Design review of the part built by this model. Coordinates are the model's own, in mm. Face numbers are marked on the shaded views. A direction names the side the tool comes from. Coordinates: 2 decimals unless noted, no trailing zeros. Write each loop counter-clockwise with the first axis right and the second up, starting at its lowest first coordinate (ties: lowest second). Pieces come first, ordered by that corner, then holes. Notation, with made-up numbers: (27, -21.75) -> (75, -21.75) arc R13 cw to (75, -11.75) -> close; hole circle Ø7 at (0, -40). An arc over 180 degrees is marked (long way). Answer in a Markdown table with one row per item. Add a question column.
Item 1: Take a section at B-B, the plane y = -6. Write out the cut boundary in (x, z), and give its area (3 significant figures).
Item 2: For the marked faces 1, 2, 3 and 4, list the 3-axis set-ups (+Z, -Z, +X, -X, +Y, -Y) from which the entire face can be reached by the end or side of a thin tool; tool diameter is ignored.
Item 3: Take a section at D-D, the plane z = 2. Write out the cut boundary in (x, y), and give its area (3 significant figures).
Item 4: Clearance check with flat-ended pins moving along their axes: P1, Ø3.5, axis at y = -15, z = -3.5, coming from the +X side; P2, Ø2, axis at x = -10, z = -6.5, coming from the +Y side; P3, Ø4, axis at y = -0.5, z = 0.5, coming from the +X side. State where each tip first meets the part, or that it passes through.
Item 5: To check wall thickness, follow line 1 (Z direction, x = -5.5, y = -11); line 2 (Y direction, x = -10, z = -5.75); line 3 (Y direction, x = 2.25, z = -8). State the ranges of each line that lie inside material, in increasing order.
Item 6: Take a section at C-C, the plane y = -12.5. Write out the cut boundary in (x, z), and give its area (3 significant figures).
Item 7: Draft analysis for pull direction Y (two halves, no side actions). For the marked faces 5, 6 and 7, state which applies: released by +Y, released by -Y, zero draft, split by the parting line, or undercut.
Item 8: Take a section at A-A, the plane z = -3. Write out the cut boundary in (x, y), and give its area (3 significant figures).
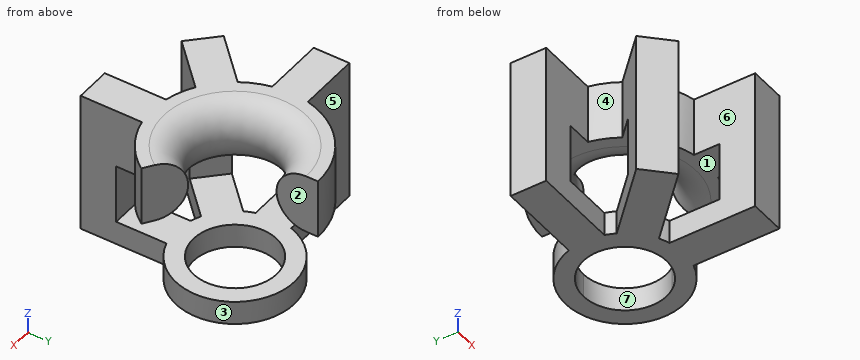
Autodesk Fusion 360 part; units mm, degrees
sketch "Sketch1" plane through (0, 0, 0) normal (1, 0, 0) x (0, 1, 0)
  line L0 (0, -2.5) -> (1, -2.5)
  line L1 (1, -2.5) -> (1, 2.5)
  line L2 (1, 2.5) -> (0, 2.5)
  arc A0 (0, 2.5) -> (0, -2.5) centre (0, 0) ccw
  line L3 (-6, 5) -> (-6, -5)
  dimension "d1" = 5
  dimension "d2" = 1
  dimension "d3" = 5
  dimension "d4" = 6
revolve "Revolve1" add sketch "Sketch1" angle 235 about axis through (0, -6, 5) along (0, 0, 1) makes body 1
sketch "Sketch2" plane through (0, 0, 2.5) normal (0, 0, 1) x (-1, 0, 0)
  line L0 (0, 0) -> (0, -1)
  arc A0 (0, -1) -> (-5.7341, 10.015) centre (0, 6) ccw
  line L1 (-5.7341, 10.015) -> (-4.9149, 9.4415)
  arc A1 (0, 0) -> (-4.9149, 9.4415) centre (0, 6) ccw
  line L2 (6, 7.5) -> (12, 7.5)
  line L3 (12, 7.5) -> (12, 4.5)
  line L4 (12, 4.5) -> (6, 4.5)
  line L5 (6, 4.5) -> (6, 7.5)
  line L6 (12, 7.5) -> (9, 7.5)
  line L7 (9, 7.5) -> (9, 4.5)
  line L8 (9, 4.5) -> (12, 4.5)
  line L9 (12, 4.5) -> (12, 7.5)
  line L10 (7.4246, 15.5459) -> (5.3033, 13.4246)
  line L11 (5.3033, 13.4246) -> (7.4246, 11.3033)
  line L12 (9.5459, 13.4246) -> (7.4246, 15.5459)
  line L13 (7.4246, 11.3033) -> (9.5459, 13.4246)
  line L14 (7.4246, 15.5459) -> (9.5459, 13.4246)
  line L15 (5.3033, 9.182) -> (3.182, 11.3033)
  line L16 (3.182, 11.3033) -> (7.4246, 15.5459)
  line L17 (9.5459, 13.4246) -> (5.3033, 9.182)
  line L18 (-1.5, 18) -> (-1.5, 15)
  line L19 (-1.5, 15) -> (1.5, 15)
  line L20 (1.5, 18) -> (-1.5, 18)
  line L21 (1.5, 15) -> (1.5, 18)
  line L22 (-1.5, 18) -> (1.5, 18)
  line L23 (1.5, 12) -> (-1.5, 12)
  line L24 (-1.5, 12) -> (-1.5, 18)
  line L25 (1.5, 18) -> (1.5, 12)
  dimension "d6" = 6
  dimension "d7" = 3
  dimension "d8" = 12
  dimension "d9" = 1.5
  dimension "d10" = 3
  dimension "d11" = 3
  dimension "d13" = 90
extrude "Extrude1" add sketch "Sketch2" against normal blind 12 separate body contours L2 L3 L4 L6 L7 L8 L9 | L10 L11 L12 L13 L14 L16 L17 | L18 L19 L20 L21 L22 L24 L25 makes body 2 at (-6.0104, -14.1317, -5.5) makes body 3 at (0.5, -15, -1.5) makes body 4 at (-9, -6.5, -1.5)
extrude "Extrude2" add sketch "Sketch2" against normal blind 5 contours A0 L2 L4 L7 | A0 L11 L16 L17 | A0 L19 L24 L25 bodies 1 2 3 4
sketch "Sketch3" plane through (0, 0, -9.5) normal (0, 0, -1) x (1, 0, 0)
  line L0 (-1.5, 15) -> (1.5, 15)
  line L1 (1.5, 15) -> (1.5, 18)
  line L2 (1.5, 18) -> (-1.5, 18)
  line L3 (-1.5, 18) -> (-1.5, 15)
  line L4 (-12, 7.5) -> (-6.8374, 7.5)
  line L5 (-6.8374, 4.5) -> (-12, 4.5)
  line L6 (-12, 4.5) -> (-12, 7.5)
  arc A0 (-6.8374, 4.5) -> (0, -1) centre (0, 6) ccw
  line L7 (-1.5, 18) -> (-1.5, 12.8374)
  line L8 (1.5, 18) -> (-1.5, 18)
  line L9 (1.5, 12.8374) -> (1.5, 18)
  arc A1 (-1.5, 12.8374) -> (-3.7741, 11.8954) centre (0, 6) ccw
  line L10 (-9.5459, 13.4246) -> (-5.8954, 9.7741)
  line L11 (-7.4246, 15.5459) -> (-9.5459, 13.4246)
  line L12 (-3.7741, 11.8954) -> (-7.4246, 15.5459)
  arc A2 (-5.8954, 9.7741) -> (-6.8374, 7.5) centre (0, 6) ccw
  arc A3 (5.7341, 10.015) -> (1.5, 12.8374) centre (0, 6) ccw
  line L13 (0, -1) -> (0, 0)
  line L14 (4.9149, 9.4415) -> (5.7341, 10.015)
  line L15 (0, 0) -> (0, 2.5)
  line L16 (2.867, 8.0075) -> (4.9149, 9.4415)
  arc A4 (2.867, 8.0075) -> (0, 2.5) centre (0, 6) ccw
  circle A5 centre (0, 6) radius 3.5
  circle A6 centre (0, 6) radius 5
  line L17 (1.5, 12.8374) -> (-1.5, 12.8374)
  line L18 (-1.5, 12.8374) -> (-1.5, 9.8374)
  line L19 (-1.5, 9.8374) -> (1.5, 9.8374)
  line L20 (1.5, 9.8374) -> (1.5, 12.8374)
  line L21 (-3.7741, 7.6528) -> (-1.6528, 9.7741)
  line L22 (-1.6528, 9.7741) -> (-3.7741, 11.8954)
  line L23 (-5.8954, 9.7741) -> (-3.7741, 7.6528)
  line L24 (-3.7741, 11.8954) -> (-5.8954, 9.7741)
  line L25 (-3.8374, 4.5) -> (-3.8374, 7.5)
  line L26 (-3.8374, 7.5) -> (-6.8374, 7.5)
  line L27 (-6.8374, 4.5) -> (-3.8374, 4.5)
  line L28 (-6.8374, 7.5) -> (-6.8374, 4.5)
  dimension "d18" = 7
  dimension "d19" = 10
  dimension "d20" = 3
  dimension "d21" = 3
  dimension "d23" = 90
extrude "Extrude3" add sketch "Sketch3" against normal blind 2 contours L0 L7 L9 L17 | A6 L17 L18 L20 | L10 L11 L12 L24 | A6 L22 L23 L24 | L15 L16 A4 A5 A6 L18 L19 L20 L21 L22 L23 L25 L26 L27 | A6 L18 L19 L20 | A6 L21 L22 L23 | L15 L16 A5 A6 | L4 L5 L6 L28 | A6 L26 L27 L28 | A6 L25 L26 L27 bodies 1
Answers:
| question | item | result |
|---|---|---|
| 1 | outline | (-12, -9.5) -> (-3.5, -9.5) -> (-3.5, -7.5) -> (-9, -7.5) -> (-9, -2.5) -> (-6, -2.5) arc R2.5 ccw to (-6, 2.5) -> (-12, 2.5) -> close; (3.5, -9.5) -> (5, -9.5) -> (5, -7.5) -> (3.5, -7.5) -> close |
| 1 | area | 74.8 mm^2 |
| 2 | face 1 | +X, +Y |
| 2 | face 2 | +Z, +X, +Y |
| 2 | face 3 | -Z |
| 2 | face 4 | +Z, -Z, -X |
| 3 | outline | (-12, -7.5) -> (-6.84, -7.5) arc R7 ccw to (-5.9, -9.77) -> (-9.55, -13.42) -> (-7.42, -15.55) -> (-3.77, -11.9) arc R7 ccw to (-1.5, -12.84) -> (-1.5, -18) -> (1.5, -18) -> (1.5, -12.84) arc R7 ccw to (5.73, -10.02) -> (3.69, -8.58) arc R4.5 cw (long way) to (0, -1.5) -> (0, 1) arc R7 ccw to (-6.84, -4.5) -> (-12, -4.5) -> close |
| 3 | area | 104 mm^2 |
| 4 | P1 | stops at x = 1.5 |
| 4 | P2 | stops at y = -4.5 |
| 4 | P3 | stops at x = 0 |
| 5 | line 1 | z = -9.5 to -7.5, -2.5 to 2.5 |
| 5 | line 2 | y = -7.5 to -4.5 |
| 5 | line 3 | y = -10.47 to -8.68, -3.32 to -1.53 |
| 6 | outline | (-8.62, -9.5) -> (-4.38, -9.5) -> (-4.38, -7.5) -> (-6.23, -7.5) -> (-6.23, -2.5) -> (-4.38, -2.5) -> (-4.38, 2.5) -> (-8.62, 2.5) -> close; (-2.6, -2.5) -> (2.6, -2.5) -> (2.6, 2.5) -> (-2.6, 2.5) -> close; (-1.5, -9.5) -> (1.5, -9.5) -> (1.5, -7.5) -> (-1.5, -7.5) -> close |
| 6 | area | 73.6 mm^2 |
| 7 | face 5 | released by +Y |
| 7 | face 6 | zero draft |
| 7 | face 7 | undercut |
| 8 | outline | (-12, -7.5) -> (-9, -7.5) -> (-9, -4.5) -> (-12, -4.5) -> close; (-9.55, -13.42) -> (-7.42, -15.55) -> (-5.3, -13.42) -> (-7.42, -11.3) -> close; (-1.5, -18) -> (1.5, -18) -> (1.5, -15) -> (-1.5, -15) -> close |
| 8 | area | 27.0 mm^2 |
